The model under review builds one solid part; all positions refer to its coordinate system, in mm. Face numbers are marked on the shaded views. A direction names the side the tool comes from. Round coordinates to 2 decimals unless told otherwise and drop trailing zeros. Order: outer loops, then holes, each group sorted by start corner. A loop starts at its lowest first (then second) coordinate and runs counter-clockwise, first axis right, second up. Notation, with made-up numbers: (80.5, 86) -> (85.5, 86) arc R20 cw to (85.5, 117) -> close; hole circle Ø5 at (-38, -8). An arc over 180 degrees is marked (long way). Use a Markdown table: item, result. Add a question column.
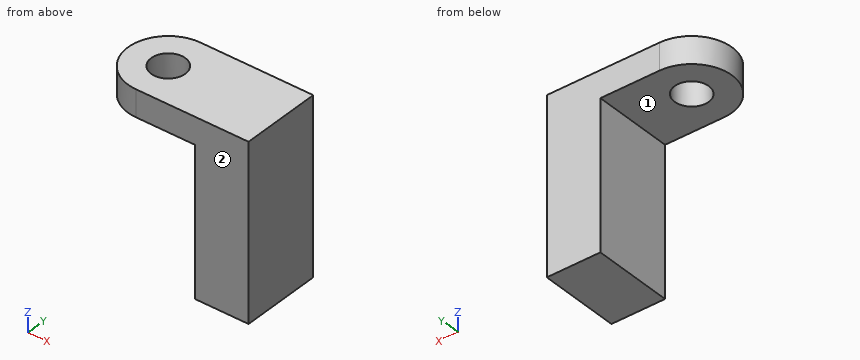
```python
from build123d import *

# Parameters (mm, degrees)
SKETCH1_W           = 20
SKETCH1_H           = 30
BOSS_EXTRUDE1_DEPTH = 55
BOSS_EXTRUDE2_DEPTH = 10
SKETCH3_R           = 6.35
CUT_EXTRUDE1_DEPTH  = 10


with BuildPart() as part:
    # Sketch1 → Boss-Extrude1 (new body)
    with BuildSketch(Plane.XY):
        with Locations((32, 0)):
            Rectangle(SKETCH1_W, SKETCH1_H)
    extrude(amount=BOSS_EXTRUDE1_DEPTH)

    # Sketch2 → Boss-Extrude2 (add)
    with BuildSketch(Plane.XY.offset(55)):
        with BuildLine():
            Line((42, 15), (42, -15))
            Line((42, -15), (0, -15))
            ThreePointArc((0, -15), (-15, 0), (0, 15))
            Line((0, 15), (42, 15))
        make_face()
    extrude(amount=BOSS_EXTRUDE2_DEPTH)

    # Sketch3 → Cut-Extrude1 (cut)
    with BuildSketch(Plane.XY.offset(65)):
        Circle(SKETCH3_R)
    extrude(amount=-CUT_EXTRUDE1_DEPTH, mode=Mode.SUBTRACT)


solid = part.part
```
Q1. For pin 1 (1 mm diameter, centred on y = 4, z = 42, fed in from -X); pin 2 (5 mm diameter, centred on x = 17.5, y = -1, fed in from -Z), all flat-tipped, find the tip position at first contact; note any pin that passes through.
Q2. To check wall thickness, follow line 1 along Y through (x, z) = (0, 62); line 2 along Z through (x, y) = (16.5, -3.25); line 3 along X through (y, z) = (5.25, 25). State the ranges of each line that lie inside material, in increasing order.
Q3. Add section C-C, the plane z = 60. Give the boundary of the cut face in (x, y), then the cut area to 3 significant figures.
Q4. Add section D-D, the plane y = -4.75. Give the boundary of the cut face in (x, z).
Q5. Add section B-B, the plane x = -2. Give the boundary of the cut face in (y, z).
Q6. Add section A-A, the plane y = 0. Give the boundary of the cut face in (x, z), then the cut area to 3 significant figures.
Q7. For the marked faces 1 and 2, list the 3-axis set-ups (+Z, -Z, +X, -X, +Y, -Y) from which the entire face can be reached by the end or side of a thin tool; tool diameter is ignored.
Return value:
| question | item | result |
|---|---|---|
| 1 | pin 1 | x = 22 |
| 1 | pin 2 | z = 55 |
| 2 | line 1 | -15 to -6.35, 6.35 to 15 |
| 2 | line 2 | 55 to 65 |
| 2 | line 3 | 22 to 42 |
| 3 | outline | (0, -15) -> (42, -15) -> (42, 15) -> (0, 15) arc R15 ccw to start; hole circle Ø12.7 at (0, 0) |
| 3 | area | 1,490 mm² |
| 4 | outline | (-14.23, 55) -> (-4.21, 55) -> (-4.21, 65) -> (-14.23, 65) -> close; (4.21, 55) -> (22, 55) -> (22, 0) -> (42, 0) -> (42, 65) -> (4.21, 65) -> close |
| 5 | outline | (-14.87, 55) -> (-6.03, 55) -> (-6.03, 65) -> (-14.87, 65) -> close; (6.03, 55) -> (14.87, 55) -> (14.87, 65) -> (6.03, 65) -> close |
| 6 | outline | (-15, 55) -> (-6.35, 55) -> (-6.35, 65) -> (-15, 65) -> close; (6.35, 55) -> (22, 55) -> (22, 0) -> (42, 0) -> (42, 65) -> (6.35, 65) -> close |
| 6 | area | 1,540 mm² |
| 7 | face 1 | -Z, -X, +Y, -Y |
| 7 | face 2 | +Z, -Z, +X, -X, -Y |
